```python
from build123d import *

# Parameters (mm, degrees)
BOSS_EXTRUDE1_DEPTH  = 12.7
M5_CLEARANCE_HOLE2_D = 5.5


with BuildPart() as part:
    # Sketch1 → Boss-Extrude1 (new body)
    with BuildSketch(Plane.XY):
        with BuildLine():
            Line((25.4, 0), (38.1, 0))
            Line((38.1, 0), (38.1, 3.175))
            Line((38.1, 3.175), (28.030256121, 3.175))
            ThreePointArc((28.030256121, 3.175), (19.05, 9.525), (10.069743879, 3.175))
            Line((10.069743879, 3.175), (0, 3.175))
            Line((0, 3.175), (0, 0))
            Line((0, 0), (12.7, 0))
            ThreePointArc((12.7, 0), (19.05, 6.35), (25.4, 0))
        make_face()
    extrude(amount=BOSS_EXTRUDE1_DEPTH)

    # M5 Clearance Hole2 (through all)
    with Locations(Plane(origin=(0, 3.175, 0), x_dir=(1, 0, 0), z_dir=(0, 1, 0))):
        with Locations((4.7625, -6.35), (33.3375, -6.35)):
            Hole(M5_CLEARANCE_HOLE2_D / 2)


solid = part.part
```
Verification items for the finished model (mm, model axes). A direction names the side the tool comes from. Coordinates: 2 decimals unless noted, no trailing zeros. Write each loop counter-clockwise with the first axis right and the second up, starting at its lowest first coordinate (ties: lowest second). Pieces come first, ordered by that corner, then holes. Notation, with made-up numbers: M -15,62.25 L 15,62.25 A20 ccw 15,71.25 Z; hole C 50.5,48 d11. An arc over 180 degrees is marked long. Answer as a JSON object with one key per item and string values. Group by question number.
(1) Material ranges on line 1 (X direction, y = 1, z = 8.25); line 2 (X direction, y = 5.25, z = 1.25); line 3 (Y direction, x = 34.5, z = 9.25) (3 decimals), recorded low to high.
(2) Cross-section at D-D, the plane x = 6.5. Record the cut outline in (y, z) (3 decimals).
(3) Cross-section at A-A, the plane z = 6.35. State how many separate pieces and enclosed holes the cut face has, and give its area (3 significant figures).
(4) Cross-section at C-C, the plane x = 28.5. Record the cut outline in (y, z) (3 decimals), and give its area (3 significant figures).
(5) Cross-section at B-B, the plane x = 32.5. Record the cut outline in (y, z) (3 decimals), and give its area (3 significant figures).
(6) Tool access check on faces 1 (the face through (33, 3.175, 3)), 2 (the face through (30, 0, 6)), 3 (the face through (7.3, 3.175, 4.8)). Record the directions out of +Z, -Z, +X, -X, +Y, -Y that give a thin tool (end or side, any length) a straight path to the whole face; none if there is none.
(7) Gauge pin test, flat ends, axial feed: pin 1 (2 mm diameter, centred on y = 7, z = 5, fed in from -X); pin 2 (5 mm diameter, centred on x = 5.5, z = 7, fed in from +Y) (3 decimals); pin 3 (4 mm diameter, centred on x = 12.5, y = 6, fed in from -Z). Record the tip position at first contact, or that the pin passes through.
(8) Release check for a two-part mould opening along X. For faces 4 (the face through (19, 7, 12.7)), 5 (the face through (38.1, 2, 6)), 6 (the face through (18.91, 6.35, 6.26)) record: +X half, -X half, draft (parallel to the pull), parting line (faces both ways), or undercut.
Reply:
{
 "1": {"line 1": "0 to 2.77, 6.75 to 12.78, 25.32 to 31.35, 35.33 to 38.1", "line 2": "11.1 to 15.48, 22.62 to 27", "line 3": "0 to 3.175"},
 "2": {"outline": "M 0,0 L 3.175,0 L 3.175,4.218 L 0,4.218 Z; M 0,8.482 L 3.175,8.482 L 3.175,12.7 L 0,12.7 Z"},
 "3": {"separate pieces": "3", "enclosed holes": "0", "area": "106 mm²"},
 "4": {"outline": "M 0,0 L 3.175,0 L 3.175,12.7 L 0,12.7 Z", "area": "40.3 mm²"},
 "5": {"outline": "M 0,0 L 3.175,0 L 3.175,3.731 L 0,3.731 Z; M 0,8.969 L 3.175,8.969 L 3.175,12.7 L 0,12.7 Z", "area": "23.7 mm²"},
 "6": {"face 1": "+Z, -Z, +X, +Y", "face 2": "+Z, -Z, +X, -X, -Y", "face 3": "+Z, -Z, -X, +Y"},
 "7": {"pin 1": "x = 11.65", "pin 2": "y = 3.175", "pin 3": "z = 0"},
 "8": {"face 4": "draft", "face 5": "+X half", "face 6": "undercut"}
}
